```python
from build123d import *

# Parameters (mm, degrees)
SKETCH2_R           = 3.189369039
SKETCH2_R_2         = 2.589261351
BOSS_EXTRUDE1_DEPTH = 10
SKETCH3_R           = 2.849023425
BOSS_EXTRUDE2_DEPTH = 1
FILLET1_R           = 1
SWEEP1_PITCH        = 3


with BuildPart() as part:
    # Sketch2 → Boss-Extrude1 (new body)
    with BuildSketch(Plane(origin=(0, 0, 0), x_dir=(0, 0, -1), z_dir=(1, 0, 0))):
        Circle(SKETCH2_R)
        Circle(SKETCH2_R_2, mode=Mode.SUBTRACT)
    extrude(amount=BOSS_EXTRUDE1_DEPTH)

    # Sketch3 → Boss-Extrude2 (add)
    with BuildSketch(Plane(origin=(10, 0, 0), x_dir=(0, 0, -1), z_dir=(1, 0, 0))):
        Circle(SKETCH3_R)
    extrude(amount=BOSS_EXTRUDE2_DEPTH)

    # Fillet1
    fillet1_edges = [part.edges().sort_by_distance(p)[0] for p in [
        (11, 0, 2.849023425),
    ]]
    fillet(fillet1_edges, radius=FILLET1_R - 0.0001)  # a hair under: the kernel refuses the full size

    # Sweep1: the profile of Sketch7 profile screwed along a right-hand helix of 3.1 turns, 10 arcs to a turn; built about Z, then put on its axis
    sweep1_z = Axis((0, 0, 0), (0, 0, 1))
    sweep1_corners = [(2.589561351, 0, -0.0003), (2.589561351, 0, 1.5003), (2.289261351, 0, 1.2), (2.289261351, 0, 0.3)]
    with BuildLine(mode=Mode.PRIVATE) as sweep1_profile:
        Line(sweep1_corners[0], sweep1_corners[1])
        Line(sweep1_corners[1], sweep1_corners[2])
        Line(sweep1_corners[2], sweep1_corners[3])
        Line(sweep1_corners[3], sweep1_corners[0])
    sweep1_cap = Face(sweep1_profile.wire())
    sweep1_turn_angles = [0, 18, 36, 54, 72, 90, 108, 126, 144, 162, 180, 198, 216, 234, 252, 270, 288, 306, 324, 342, 360]
    sweep1_turn_weights = [1, 0.9510565162951535, 1, 0.9510565162951535, 1, 0.9510565162951535, 1, 0.9510565162951535, 1, 0.9510565162951535, 1, 0.9510565162951535, 1, 0.9510565162951535, 1, 0.9510565162951535, 1, 0.9510565162951535, 1, 0.9510565162951535, 1]
    sweep1_turn_rails = [Edge.make_bspline([Vector(p[0], p[1], 0).rotate(sweep1_z, sweep1_turn_angles[k]) / sweep1_turn_weights[k] + Vector(0, 0, p[2] + SWEEP1_PITCH * sweep1_turn_angles[k] / 360) for k in range(21)], [0, 0, 0, 1, 1, 2, 2, 3, 3, 4, 4, 5, 5, 6, 6, 7, 7, 8, 8, 9, 9, 10, 10, 10], 2, sweep1_turn_weights) for p in sweep1_corners]
    sweep1_turn_sides = [Face.make_surface_from_curves(sweep1_turn_rails[p[0]], sweep1_turn_rails[p[1]]) for p in [(0, 1), (1, 2), (2, 3), (3, 0)]]
    sweep1_last_angles = [1080, 1098, 1116]
    sweep1_last_weights = [1, 0.9510565162951499, 1]
    sweep1_last_rails = [Edge.make_bspline([Vector(p[0], p[1], 0).rotate(sweep1_z, sweep1_last_angles[k]) / sweep1_last_weights[k] + Vector(0, 0, p[2] + SWEEP1_PITCH * sweep1_last_angles[k] / 360) for k in range(3)], [0, 0, 0, 1, 1, 1], 2, sweep1_last_weights) for p in sweep1_corners]
    sweep1_last_sides = [Face.make_surface_from_curves(sweep1_last_rails[p[0]], sweep1_last_rails[p[1]]) for p in [(0, 1), (1, 2), (2, 3), (3, 0)]]
    sweep1 = Plane(origin=(0, 0, 0), x_dir=(0, 0, 1), z_dir=(1, 0, 0)) * Solid(Shell([*[p.moved(Location((0, 0, SWEEP1_PITCH * i))) for i in range(3) for p in sweep1_turn_sides], *sweep1_last_sides, sweep1_cap, sweep1_cap.rotate(sweep1_z, 1116).moved(Location((0, 0, SWEEP1_PITCH * 1116 / 360)))]))
    add(sweep1)


solid = part.part
```
Source: CAD feature listing. Evaluate the final solid. Frame: model axes, mm. A direction names the side the tool comes from. Round coordinates to 2 decimals unless told otherwise and drop trailing zeros. Use a Markdown table: item, result. Add a question column.
1. Set-up query: faces 4 (the flat face through (0, 3, 0)), 5 (the flat face through (10, 3, 0)). Return all of +Z, -Z, +X, -X, +Y, -Y with unobstructed straight access to the full face (end or side cutting, diameter ignored); none if empty.
2. Contact query for flat-ended pins moving along their axis: pin 1 (3 mm diameter, centred on y = 1, z = -1.5, fed in from -X); pin 2 (1 mm diameter, centred on x = 6, y = -1, fed in from -Z); pin 3 (3 mm diameter, centred on y = 0, z = 0, fed in from -X); pin 4 (1.5 mm diameter, centred on x = 8.5, y = 1, fed in from +Z). Output: stop coordinate, or through.
3. Ray query, line 1 along Y through (x, z) = (9, 0); line 2 along Y through (x, z) = (7.7, 0); line 3 along X through (y, z) = (-2.5, -0.5). Return the intervals inside material, ascending. Write a range as [from, to].
4. Pull-direction query (Y, two-part tool) for faces 1 (the cylindrical face through (4.93, -1.222, -2.946)), 2 (the flat face through (11, 0, 0)), 3 (the flat face through (10, 0, 0)); classes: +Y half, -Y half, draft (parallel to the pull), parting line (faces both ways), or undercut.
Solution:
| question | item | result |
|---|---|---|
| 1 | face 4 | +Z, -Z, -X, +Y, -Y |
| 1 | face 5 | +X |
| 2 | pin 1 | stops at x = 0 |
| 2 | pin 2 | stops at z = -3.15 |
| 2 | pin 3 | stops at x = 10 |
| 2 | pin 4 | stops at z = 3.18 |
| 3 | line 1 | y = [-3.19, -2.59], [2.29, 3.19] |
| 3 | line 2 | y = [-3.19, -2.29], [2.59, 3.19] |
| 3 | line 3 | x = [0.88, 2.31], [3.88, 5.31], [6.88, 8.31], [10, 10.71] |
| 4 | face 1 | parting line |
| 4 | face 2 | draft |
| 4 | face 3 | undercut |
